The drawing under review shows one solid part. Ordinate dimensions are in mm from its lowest x, y, z. A direction names the side the tool comes from. Give positions to 0.01 mm unless a question says otherwise; leave off trailing zeros. Loops run counter-clockwise (first coordinate to the right, second up) from the corner with the lowest first, then second, coordinate; pieces in that order, holes last. Notation, with made-up numbers: (-39, -39.75) - (-29, -39.75) arc R15 ccw to (-29, -13.75) - close; hole circle Ø7 at (54.5, -29). An arc over 180 degrees is marked (long way). Write each question's results on one line, items separated by ' | '.
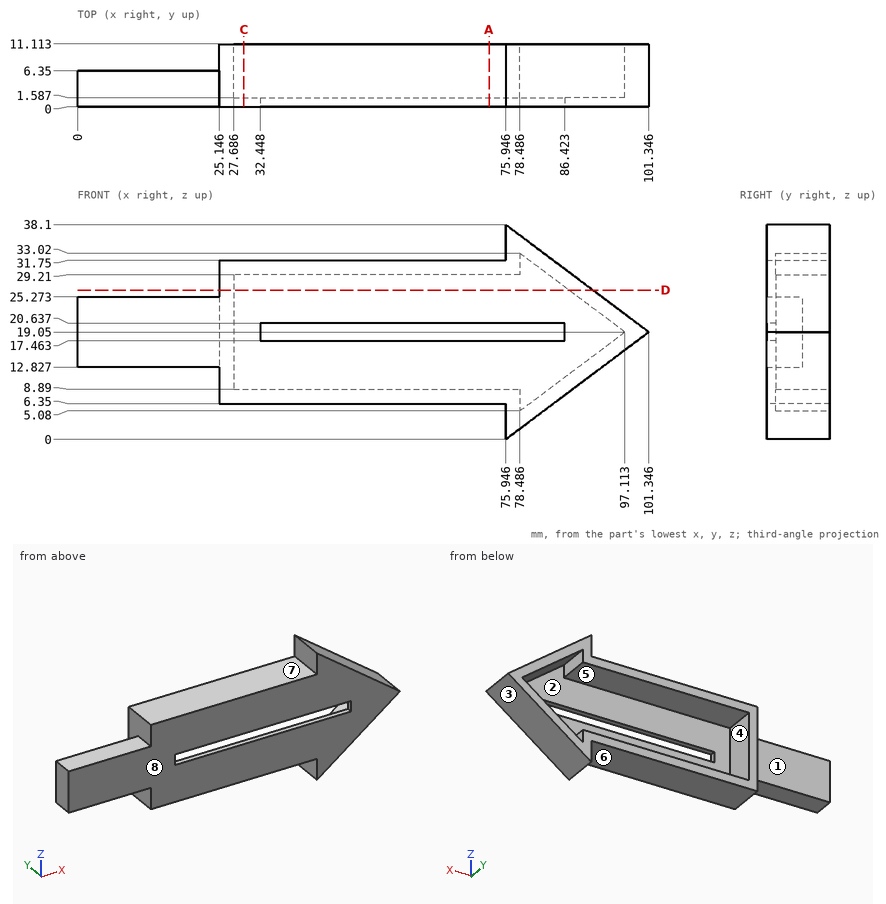
(1) Wall thickness on line 1 along Z through (x, y) = (29, 7.25); line 2 along Y through (x, z) = (43, 11.5); line 3 along X through (y, z) = (6, 25.5) (1 decimal): over which ranges is each line inside the solid? List them lowest first. Write a range as from..to.
Answers below:
line 1: 6.35..8.89, 29.21..31.75 | line 2: 0..1.59 | line 3: 25.1..27.7, 88.5..92.7
(2) Draft analysis for pull direction X (two halves, no side actions). For the marked faces 1, 2, 3 and 4, state which applies: pulls with the +X half, pulls with the -X half, needs draft (parallel to the pull), parting line crosses it, or undercut.
Answers below:
face 1: needs draft | face 2: undercut | face 3: pulls with the +X half | face 4: undercut
(3) Take a section at D-D on z = 26.5. Give the boundary of the cut face in (x, y) (1 decimal), plus the area to 3 significant figures.
Answers below:
outline: (25.1, 0) - (91.4, 0) - (91.4, 11.1) - (87.2, 11.1) - (87.2, 1.6) - (27.7, 1.6) - (27.7, 11.1) - (25.1, 11.1) - close | area: 170 mm2
(4) Insertion check: P1, Ø3, axis at x = 17, y = 3, coming from the +Z side; P2, Ø5, axis at y = 6, z = 7, coming from the -X side; P3, Ø1.5, axis at x = 70, y = 7.5, coming from the +Z side. Each pin has a flat end and moves straight along its axis. Give the tip position at first contact, or say it passes through.
Answers below:
P1: z = 25.27 | P2: x = 25.15 | P3: z = 31.75
(5) Take a section at A-A on x = 73. Give the boundary of the cut face in (y, z).
Answers below:
outline: (0, 6.35) - (11.11, 6.35) - (11.11, 8.89) - (1.59, 8.89) - (1.59, 17.46) - (0, 17.46) - close; (0, 20.64) - (1.59, 20.64) - (1.59, 29.21) - (11.11, 29.21) - (11.11, 31.75) - (0, 31.75) - close
(6) Tool access review of the marked faces 5, 6, 7 and 8: name each direction out of +Z, -Z, +X, -X, +Y, -Y from which nothing blocks a thin tool from reaching the whole face with its end or side.
Answers below:
face 5: +Y | face 6: -Z, -X, +Y, -Y | face 7: +Z, -X, +Y, -Y | face 8: +Z, -Z, +X, -X, -Y
(7) Take a section at C-C on x = 29.5. Give the boundary of the cut face in (y, z).
Answers below:
outline: (0, 6.35) - (11.11, 6.35) - (11.11, 8.89) - (1.59, 8.89) - (1.59, 29.21) - (11.11, 29.21) - (11.11, 31.75) - (0, 31.75) - close
